Autodesk Inventor part; units mm, degrees
ref_plane "YZ Plane" through (0, 0, 0) normal (1, 0, 0) x (0, 1, 0)
ref_plane "XZ Plane" through (0, 0, 0) normal (0, 1, 0) x (-1, 0, 0)
ref_plane "XY Plane" through (0, 0, 0) normal (0, 0, 1) x (1, 0, 0)
sketch "Sketch1" plane through (0, 0, 0) normal (0, 0, 1) x (1, 0, 0)
  line L0 (0, 0) -> (0, 50.8) construction
  line L1 (0, 0) -> (50.8, 0) construction
  line L2 (31.75, 18.9992) -> (31.75, 19.1008)
  line L3 (0, 9.5479) -> (15.8115, 9.5479) construction
  line L4 (31.75, 18.9992) -> (15.875, 18.9992)
  line L5 (15.875, 18.9992) -> (15.875, 0)
  line L6 (0, 0) -> (8.2867, 0) construction
  line L7 (8.2867, 0) -> (15.875, 0)
  line L8 (8.2867, 0) -> (8.2867, 12.7)
  line L9 (4.0259, 71.0633) -> (4.0259, -11.3243) construction
  line L10 (8.2867, 12.7) -> (4.0259, 12.7)
  line L11 (4.0259, 19.1008) -> (4.0259, 12.7)
  line L12 (31.75, 36.068) -> (31.75, 19.1008)
  line L13 (31.75, 36.068) -> (0, 36.068)
  line L14 (4.0259, 19.1008) -> (0, 19.1008)
  line L15 (0, 36.068) -> (0, 19.1008)
  dimension "d12" = 15.8115
  dimension "d15" = 8.2867
  dimension "d55" = 4.0259
  dimension "d56" = 12.7
  dimension "d95" = 6.4008
revolve "Revolution1" add sketch "Sketch1" angle 360 about axis through (0, 0, 0) along (0, 1, 0)
sketch "Sketch2" plane through (0, 0, 0) normal (0, -1, 0) x (1, 0, 0)
  circle A0 centre (0, 0) radius 8.2867 construction
  line L0 (-2.2055, 7.9879) -> (-2.2121, 9.8928)
  circle A1 centre (0, 0) radius 10.1371 construction
  line L1 (2.1506, 8.0028) -> (2.144, 9.9078)
  line L2 (-2.2055, 7.9879) -> (2.1506, 8.0028) construction
  arc A2 (2.144, 9.9078) -> (-2.2121, 9.8928) centre (0, 0) ccw
  arc A3 (2.1506, 8.0028) -> (-2.2055, 7.9879) centre (0, 0) ccw
  dimension "d43" = 1.905
  dimension "d44" = 4.3561
extrude "Extrusion1" cut sketch "Sketch2" against normal blind 12.7
pattern_circular "Circular Pattern2" count 6 over 360 about axis through (0, 6.35, 0) along (0, -1, 0) of "Extrusion1"
properties part number "denso-basic"
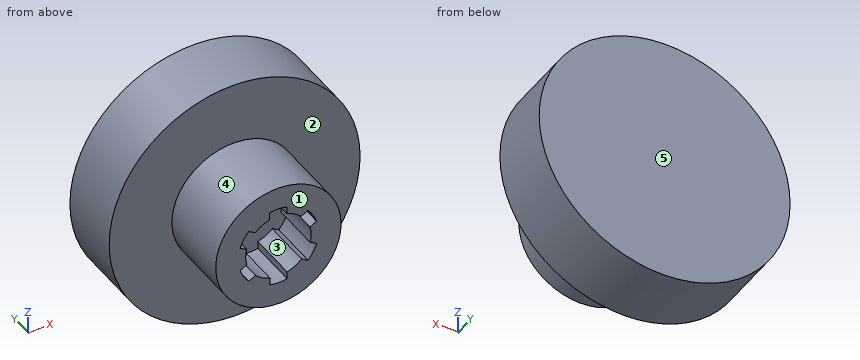
Can you work these out from the model? Positions are in its coordinate system, mm. Face numbers are marked on the shaded views. A direction names the side the tool comes from. Give positions to 0.01 mm unless a question says otherwise; leave off trailing zeros. Loops run counter-clockwise (first coordinate to the right, second up) from the corner with the lowest first, then second, coordinate; pieces in that order, holes last. Notation, with made-up numbers: M 46,22 L 84,22 A17 cw 84,44 Z; hole C 77,-18 d2. An arc over 180 degrees is marked long. One line per item, written item: value.
1) I'm going to push flat-ended pins straight in: pin 1 (4 mm diameter, centred on x = -20.5, z = -23.5, fed in from -Y); pin 2 (1.5 mm diameter, centred on x = -20.5, y = 29, fed in from +Z); pin 3 (8 mm diameter, centred on x = 12.5, y = 26.5, fed in from -Z); pin 4 (12 mm diameter, centred on x = -0.5, z = -16, fed in from -Y). Where does each tip first touch, or does it pass through?
Geometry check:
pin 1: stops at y = 19
pin 2: stops at z = 24.86
pin 3: stops at z = -30.59
pin 4: stops at y = 0
2) Imagine slicing it at D-D on x = 11. Write out the boundary of the cut face in (y, z), and give its area (3 significant figures).
Geometry check:
outline: M 0,-11.45 L 19,-11.45 L 19,-29.78 L 36.07,-29.78 L 36.07,29.78 L 19,29.78 L 19,11.45 L 0,11.45 Z
area: 1,450 mm²
3) Imagine slicing it at A-A on z = 0. Write out the boundary of the cut face in (x, y) (3 decimals), and give its area (3 significant figures).
Geometry check:
outline: M -31.75,18.999 L -15.875,18.999 L -15.875,0 L -8.287,0 L -8.287,12.7 L -4.026,12.7 L -4.026,19.101 L 4.026,19.101 L 4.026,12.7 L 8.287,12.7 L 8.287,0 L 15.875,0 L 15.875,18.999 L 31.75,18.999 L 31.75,36.068 L -31.75,36.068 Z
area: 1,430 mm²
4) On a 3-axis mill with a long thin cutter (end or side, diameter ignored), from which of +Z, -Z, +X, -X, +Y, -Y can I reach the whole of each face in a straight line? I mean the marked faces 1 and 2. Say none if no direction works.
Geometry check:
face 1: +Z, -Z, +X, -X, -Y
face 2: -Y
5) Imagine slicing it at B-B on x = 0. Write out the boundary of the cut face in (y, z) (3 decimals), and give its area (3 significant figures).
Geometry check:
outline: M 0,-15.875 L 18.999,-15.875 L 18.999,-31.75 L 36.068,-31.75 L 36.068,31.75 L 18.999,31.75 L 18.999,15.875 L 0,15.875 L 0,10.137 L 12.7,10.137 L 12.7,4.026 L 19.101,4.026 L 19.101,-4.026 L 12.7,-4.026 L 12.7,-10.137 L 0,-10.137 Z
area: 1,380 mm²
6) Thinking about a two-plate mould opening in X: for the marked faces 3, 4 and 5, which applies, +X half, -X half, draft (parallel to the pull), parting line (faces both ways), or undercut?
Geometry check:
face 3: undercut
face 4: parting line
face 5: draft
7) Imagine slicing it at C-C on y = 20.5. Write out the boundary of the cut face in (x, z), and give its area (3 significant figures).
Geometry check:
outline: C 0,0 d63.5
area: 3,170 mm²
8) Please list where these lines run through material, in increasing order: line 1 (X direction, y = 17.5, z = 0) (3 decimals); line 2 (Y direction, x = -22, z = 4).
Geometry check:
line 1: x = -15.875 to -4.026, 4.026 to 15.875
line 2: y = 19 to 36.07
